Input: part model. Units: mm. Frame: model coordinates. Face numbers are marked on the shaded views. A direction names the side the tool comes from. Round coordinates to 2 decimals unless told otherwise and drop trailing zeros. Loops run counter-clockwise (first coordinate to the right, second up) from the corner with the lowest first, then second, coordinate; pieces in that order, holes last. Notation, with made-up numbers: (3.25, -13) -> (11.25, -13) arc R9 ccw to (11.25, -2) -> close; hole circle Ø4 at (72, 68.25). An arc over 180 degrees is marked (long way). One line per question, with ' | ' between items. Start each with the question number.
Q1. Cut plane B-B on y = -70.5. Return loops of the section in (x, z), and give its area (3 significant figures).
Q2. Cut plane D-D on z = 191. Return loops of the section in (x, y).
Q3. Cut plane A-A on z = 112. Return loops of the section in (x, y).
Q4. Access query for the marked faces 4 and 5. Directions: +Z, -Z, +X, -X, +Y, -Y. A direction counts if a zero-diameter tool reaches every point of the face in a straight line with its end or side. Return the directions, or none.
Q5. Mould query, pull axis X, two halves, no side actions, for the marked faces 1, 2 and 3. Classes: pulls with the +X half, pulls with the -X half, needs draft (parallel to the pull), parting line crosses it, or undercut.
Q6. Contact query for flat-ended pins moving along their axis: P1, Ø2, axis at x = 67.5, z = 88.5, coming from the -Y side; P2, Ø6, axis at x = -57.5, z = 148, coming from the -Y side; P3, Ø10, axis at x = -58.5, z = 160, coming from the -Y side; P4, Ø8, axis at x = -2.5, z = 150.5, coming from the +Y side. Output: stop coordinate, or through.
Q7. Material intervals for L1, parallel to Z at x = -42.5, y = -71.5; L2, parallel to Z at x = 31.5, y = -69; L3, parallel to Y at x = 0, z = 242, sorted ascending.
from build123d import *

# Parameters (mm, degrees)
F0_R      = 94
F1_DEPTH  = 9
F2_R      = 50
F3_DEPTH  = 74
F4_R      = 94
F5_DEPTH  = 18
F7_DEPTH  = 77
F8_R      = 50
F9_DEPTH  = 77
F10_R     = 86
F11_DEPTH = 18
F12_R     = 3
F13_DEPTH = 77
F14_R     = 50
F15_DEPTH = 77
F16_R     = 78
F17_DEPTH = 18
F18_R     = 45
F19_DEPTH = 200


with BuildPart() as f1:
    # F0 (on Top) → F1 (new body)
    with BuildSketch(Plane.XY):
        Circle(F0_R)
    extrude(amount=F1_DEPTH)

    # F2 (on face) → F3 (join)
    with BuildSketch(Plane.XY.offset(9)):
        Circle(F2_R)
    extrude(amount=F3_DEPTH)

    # F4 (on face) → F5 (join)
    with BuildSketch(Plane.XY.offset(83)):
        Circle(F4_R)
    extrude(amount=F5_DEPTH)

    # F6 (on face) → F7 (join)
    with BuildSketch(Plane.XY.offset(101)):
        with BuildLine():
            ThreePointArc((-2.9991759122, 63.9296875), (0, 61), (2.9991759122, 63.9296875))
            ThreePointArc((2.9991759122, 63.9296875), (0, 64), (-2.9991759122, 63.9296875))
        make_face()
        with BuildLine():
            ThreePointArc((-2.9991759122, 63.9296875), (0, 64), (2.9991759122, 63.9296875))
            ThreePointArc((2.9991759122, 63.9296875), (2.999793971, 63.9648413354), (3, 64))
            ThreePointArc((3, 64), (-0.0351586646, 66.999793971), (-2.9991759122, 63.9296875))
        make_face()
        with BuildLine():
            ThreePointArc((-63.9296875, -2.9991759122), (-64, 0), (-63.9296875, 2.9991759122))
            ThreePointArc((-63.9296875, 2.9991759122), (-67, 0), (-63.9296875, -2.9991759122))
        make_face()
        with BuildLine():
            ThreePointArc((-61, 0), (-61.8539644108, 2.0963137289), (-63.9296875, 2.9991759122))
            ThreePointArc((-63.9296875, 2.9991759122), (-64, 0), (-63.9296875, -2.9991759122))
            ThreePointArc((-63.9296875, -2.9991759122), (-61.8539644108, -2.0963137289), (-61, 0))
        make_face()
        with BuildLine():
            ThreePointArc((-2.9991759122, -63.9296875), (0, -64), (2.9991759122, -63.9296875))
            ThreePointArc((2.9991759122, -63.9296875), (0, -61), (-2.9991759122, -63.9296875))
        make_face()
        with BuildLine():
            ThreePointArc((3, -64), (2.999793971, -63.9648413354), (2.9991759122, -63.9296875))
            ThreePointArc((2.9991759122, -63.9296875), (0, -64), (-2.9991759122, -63.9296875))
            ThreePointArc((-2.9991759122, -63.9296875), (-0.0351586646, -66.999793971), (3, -64))
        make_face()
        with BuildLine():
            ThreePointArc((63.9296875, -2.9991759122), (63.9824194603, -1.5), (64, 0))
            ThreePointArc((64, 0), (63.9824194603, 1.5), (63.9296875, 2.9991759122))
            ThreePointArc((63.9296875, 2.9991759122), (61, 0), (63.9296875, -2.9991759122))
        make_face()
        with BuildLine():
            ThreePointArc((63.9296875, 2.9991759122), (63.9824194603, 1.5), (64, 0))
            ThreePointArc((64, 0), (63.9824194603, -1.5), (63.9296875, -2.9991759122))
            ThreePointArc((63.9296875, -2.9991759122), (66.0963137289, -2.1460355892), (67, 0))
            ThreePointArc((67, 0), (66.0963137289, 2.1460355892), (63.9296875, 2.9991759122))
        make_face()
    extrude(amount=F7_DEPTH)

    # F8 (on face) → F9 (join)
    with BuildSketch(Plane.XY.offset(101)):
        Circle(F8_R)
    extrude(amount=F9_DEPTH)

    # F10 (on face) → F11 (join)
    with BuildSketch(Plane.XY.offset(178)):
        Circle(F10_R)
    extrude(amount=F11_DEPTH)

    # F12 (on face) → F13 (join)
    with BuildSketch(Plane.XY.offset(196)):
        with Locations((-45.2548339959, 45.2548339959)):
            Circle(F12_R)
        with Locations((45.2548339959, 45.2548339959)):
            Circle(F12_R)
        with Locations((45.2548339959, -45.2548339959)):
            Circle(F12_R)
        with Locations((-45.2548339959, -45.2548339959)):
            Circle(F12_R)
    extrude(amount=F13_DEPTH)

    # F14 (on face) → F15 (join)
    with BuildSketch(Plane.XY.offset(196)):
        Circle(F14_R)
    extrude(amount=F15_DEPTH)

    # F16 (on face) → F17 (join)
    with BuildSketch(Plane.XY.offset(273)):
        Circle(F16_R)
    extrude(amount=F17_DEPTH)

    # F18 (on face) → F19 (cut)
    with BuildSketch(Plane.XY.offset(291)):
        Circle(F18_R)
    extrude(amount=-F19_DEPTH, mode=Mode.SUBTRACT)


solid = f1.part
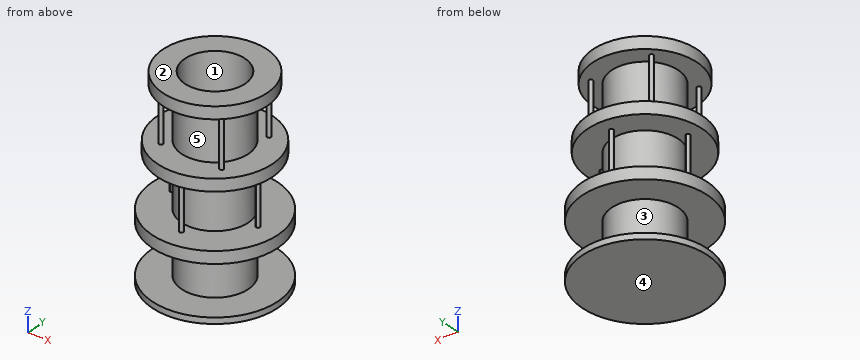
Results:
1) outline: (-62.18, 0) -> (62.18, 0) -> (62.18, 9) -> (-62.18, 9) -> close; (-62.18, 83) -> (62.18, 83) -> (62.18, 101) -> (-62.18, 101) -> close; (-49.25, 178) -> (49.25, 178) -> (49.25, 196) -> (-49.25, 196) -> close; (-33.37, 273) -> (33.37, 273) -> (33.37, 291) -> (-33.37, 291) -> close | area: 6,330 mm^2
2) outline: circle Ø172 at (0, 0); hole circle Ø90 at (0, 0)
3) outline: circle Ø6 at (-64, 0); circle Ø100 at (0, 0); circle Ø6 at (0, -64); circle Ø6 at (0, 64); circle Ø6 at (64, 0); hole circle Ø90 at (0, 0)
4) face 4: -Z, +X, -X, +Y, -Y | face 5: none
5) face 1: undercut | face 2: needs draft | face 3: parting line crosses it
6) P1: y = -66.44 | P2: through | P3: y = -2.96 | P4: y = 67
7) L1: 0 to 9, 83 to 101, 178 to 196 | L2: 0 to 9, 83 to 101, 178 to 196, 273 to 291 | L3: -50 to -45, 45 to 50
